Read the model definition and answer for the solid it produces. Units are mm, in the model's axes. Face numbers are marked on the shaded views. A direction names the side the tool comes from. Coordinates: 2 decimals unless noted, no trailing zeros. Write each loop counter-clockwise with the first axis right and the second up, starting at its lowest first coordinate (ties: lowest second). Pieces come first, ordered by that corner, then holes. Notation, with made-up numbers: (67.25, -40) -> (124.25, -40) arc R33 cw to (124.25, -7) -> close; hole circle Ø9 at (-19.75, 36). An arc over 180 degrees is marked (long way). Use CSV: the item, a comma, the result in double quotes.
from build123d import *

# Parameters (mm, degrees)
SKETCH1_W           = 14
SKETCH1_H           = 16
SKETCH1_W_2         = 10
SKETCH1_H_2         = 12
BOSS_EXTRUDE1_DEPTH = 9
SKETCH2_R           = 2.5
SKETCH2_R_2         = 0.5
BOSS_EXTRUDE2_DEPTH = 5


with BuildPart() as part:
    # Sketch1 → Boss-Extrude1 (new body)
    with BuildSketch(Plane.XY):
        with Locations((-7, 8)):
            Rectangle(SKETCH1_W, SKETCH1_H)
        with Locations((-7, 8)):
            Rectangle(SKETCH1_W_2, SKETCH1_H_2, mode=Mode.SUBTRACT)
    extrude(amount=BOSS_EXTRUDE1_DEPTH)

    # Sketch2 → Boss-Extrude2 (add)
    with BuildSketch(Plane.ZY.offset(14)):
        with Locations((4.5, 8)):
            Circle(SKETCH2_R)
        with Locations((4.5, 8)):
            Circle(SKETCH2_R_2, mode=Mode.SUBTRACT)
    extrude(amount=BOSS_EXTRUDE2_DEPTH)


solid = part.part
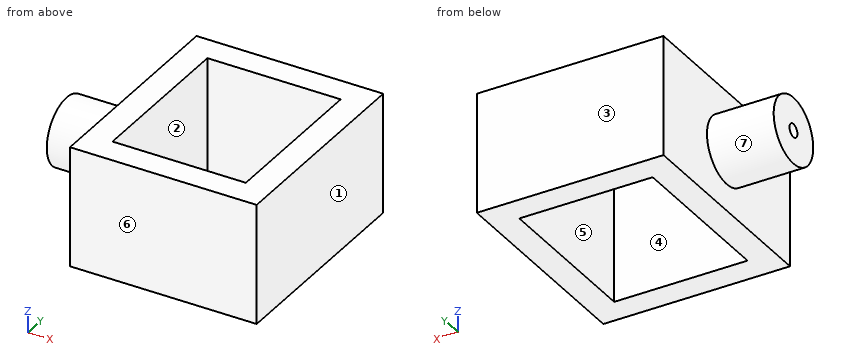
1. A cutting plane is placed at A-A (y = 4.25). Give the vertices of the cut face in (x, z), and give its area (3 significant figures).
Solutions:
outline,"(-14, 0) -> (-12, 0) -> (-12, 9) -> (-14, 9) -> close; (-2, 0) -> (0, 0) -> (0, 9) -> (-2, 9) -> close"
area,"36.0 mm^2"
2. A cutting plane is placed at C-C (x = -7.75). Give the vertices of the cut face in (y, z).
Solutions:
outline,"(0, 0) -> (2, 0) -> (2, 9) -> (0, 9) -> close; (14, 0) -> (16, 0) -> (16, 9) -> (14, 9) -> close"
3. This flat-tipped pin is pushed along its axis until it touches: pin 1 Ø5 at (y, z) = (12.5, 2) entering from -X. Where does it stop, or does it pass through?
Solutions:
pin 1,"stops at x = -14"
4. A cutting plane is placed at D-D (y = 8). Give the vertices of the cut face in (x, z), and give its area (3 significant figures).
Solutions:
outline,"(-19, 2) -> (-14, 2) -> (-14, 0) -> (-12, 0) -> (-12, 9) -> (-14, 9) -> (-14, 7) -> (-19, 7) -> (-19, 5) -> (-14, 5) -> (-14, 4) -> (-19, 4) -> close; (-2, 0) -> (0, 0) -> (0, 9) -> (-2, 9) -> close"
area,"56.0 mm^2"
5. Find the intervals of material crossed by line 1 along Y through (x, z) = (-16.05, 4.5); line 2 along X through (y, z) = (13.5, 7.75); line 3 along Y through (x, z) = (-8.25, 8.5), in increasing order.
Solutions:
line 1,"y = 5.5 to 7.5, 8.5 to 10.5"
line 2,"x = -14 to -12, -2 to 0"
line 3,"y = 0 to 2, 14 to 16"
6. For a pull along Y with two mould halves and no side action, classify the marked faces 1, 2, 3 and 4 as pulls with the +Y half, pulls with the -Y half, needs draft (parallel to the pull), parting line crosses it, or undercut.
Solutions:
face 1,"needs draft"
face 2,"undercut"
face 3,"pulls with the +Y half"
face 4,"undercut"
7. A tool of negligible diameter and unlimited length cuts with its end or side. For the marked faces 5, 6 and 7, from which of +Z, -Z, +X, -X, +Y, -Y can it reach the whole face along a straight path? Write none if from no direction.
Solutions:
face 5,"+Z, -Z"
face 6,"+Z, -Z, +X, -X, -Y"
face 7,"-X"
8. A cutting plane is placed at B-B (z = 4.5). Give the vertices of the cut face in (x, y), and give its area (3 significant figures).
Solutions:
outline,"(-19, 5.5) -> (-14, 5.5) -> (-14, 0) -> (0, 0) -> (0, 16) -> (-14, 16) -> (-14, 10.5) -> (-19, 10.5) -> (-19, 8.5) -> (-14, 8.5) -> (-14, 7.5) -> (-19, 7.5) -> close; hole (-12, 2) -> (-2, 2) -> (-2, 14) -> (-12, 14) -> close"
area,"124 mm^2"
